Read the model definition and answer for the solid it produces. Units are mm, in the model's axes. A direction names the side the tool comes from. Give positions to 0.01 mm unless a question says otherwise; leave off trailing zeros. Write each loop counter-clockwise with the first axis right and the second up, starting at its lowest first coordinate (ties: lowest second). Pieces come first, ordered by that corner, then holes. Notation, with made-up numbers: M 10.5,46.5 L 52.5,46.5 A25 ccw 52.5,63.5 Z; hole C -2,70.5 d1. An arc over 180 degrees is marked long. Put each result on its own line as item: value.
from build123d import *

# Parameters (mm, degrees)
SKETCH1_W                               = 125
SKETCH1_H                               = 100
BOSS_EXTRUDE1_DEPTH                     = 15
SKETCH2_W                               = 75.5
SKETCH2_H                               = 45.5
CUT_EXTRUDE1_DEPTH                      = 5
FILLET1_R                               = 2.5
CHAMFER2_SIZE                           = 2.5
CBORE_FOR_M5_HEX_HEAD_BOLT1_D           = 5.5
CBORE_FOR_M5_HEX_HEAD_BOLT1_CBORE_D     = 12.24
CBORE_FOR_M5_HEX_HEAD_BOLT1_CBORE_DEPTH = 3.58
LPATTERN2_COUNT                         = 2
LPATTERN2_PITCH                         = 75
LPATTERN2_COUNT_DIR2                    = 2
LPATTERN2_PITCH_DIR2                    = 100
FILLET2_R                               = 2.5
CHAMFER3_SIZE                           = 2.5


with BuildPart() as part:
    # Sketch1 → Boss-Extrude1 (new body)
    with BuildSketch(Plane(origin=(0, 0, 0), x_dir=(1, 0, 0), z_dir=(0, 1, 0))):
        Rectangle(SKETCH1_W, SKETCH1_H)
    extrude(amount=BOSS_EXTRUDE1_DEPTH)

    # Sketch2 → Cut-Extrude1 (cut)
    with BuildSketch(Plane(origin=(0, 15, 0), x_dir=(1, 0, 0), z_dir=(0, 1, 0))):
        Rectangle(SKETCH2_W, SKETCH2_H)
    extrude(amount=-CUT_EXTRUDE1_DEPTH, mode=Mode.SUBTRACT)

    # Fillet1
    fillet1_edges = [part.edges().sort_by_distance(p)[0] for p in [
        (37.75, 12.5, -22.75),
        (37.75, 12.5, 22.75),
        (-37.75, 12.5, 22.75),
        (-37.75, 12.5, -22.75),
    ]]
    fillet(fillet1_edges, radius=FILLET1_R)

    # Chamfer2
    chamfer2_edges = [part.edges().sort_by_distance(p)[0] for p in [
        (0, 15, 22.75),
        (-37.75, 15, 0),
        (37.75, 15, 0),
        (0, 15, -22.75),
        (-37.017766953, 15, 22.017766953),
        (37.017766953, 15, 22.017766953),
        (37.017766953, 15, -22.017766953),
        (-37.017766953, 15, -22.017766953),
    ]]
    chamfer(chamfer2_edges, length=CHAMFER2_SIZE)

    # CBORE for M5 Hex Head Bolt1 (through all)
    with Locations(Plane(origin=(0, 15, 0), x_dir=(1, 0, 0), z_dir=(0, 1, 0))):
        with Locations((50, 37.5)):
            cbore_for_m5_hex_head_bolt1 = CounterBoreHole(CBORE_FOR_M5_HEX_HEAD_BOLT1_D / 2, CBORE_FOR_M5_HEX_HEAD_BOLT1_CBORE_D / 2, CBORE_FOR_M5_HEX_HEAD_BOLT1_CBORE_DEPTH)

    # LPattern2: CBORE for M5 Hex Head Bolt1 2 × 2
    with Locations(*[(-j * LPATTERN2_PITCH_DIR2, 0, i * LPATTERN2_PITCH) for i in range(LPATTERN2_COUNT) for j in range(LPATTERN2_COUNT_DIR2) if (i, j) != (0, 0)]):
        add(cbore_for_m5_hex_head_bolt1, mode=Mode.SUBTRACT)

    # Fillet2
    fillet2_edges = [part.edges().sort_by_distance(p)[0] for p in [
        (62.5, 7.5, 50),
        (-62.5, 7.5, 50),
        (-62.5, 7.5, -50),
        (62.5, 7.5, -50),
    ]]
    fillet(fillet2_edges, radius=FILLET2_R)

    # Chamfer3
    chamfer3_edges = [part.edges().sort_by_distance(p)[0] for p in [
        (-62.5, 15, 0),
        (0, 15, -50),
        (62.5, 15, 0),
        (0, 15, 50),
        (-61.767766953, 15, 49.267766953),
        (61.767766953, 15, 49.267766953),
        (61.767766953, 15, -49.267766953),
        (-61.767766953, 15, -49.267766953),
    ]]
    chamfer(chamfer3_edges, length=CHAMFER3_SIZE - 0.0001)  # a hair under: the kernel refuses the full size


solid = part.part
(1) For a pull along X with two mould halves and no side action, classify faces 3 (the face through (38.98, 13.73, 0.28)), 4 (the face through (-60.89, 13.73, 48.41)), 5 (the face through (60.89, 13.73, -48.41)) as +X half, -X half, draft (parallel to the pull), parting line (faces both ways), or undercut.
Result:
face 3: undercut
face 4: -X half
face 5: +X half
(2) Section A-A on z = 37.5 is taken. Determine the outline of the cut face in (x, y), and give its area (3 significant figures).
Result:
outline: M -62.5,0 L -52.75,0 L -52.75,11.42 L -56.12,11.42 L -56.12,15 L -60,15 L -62.5,12.5 Z; M -47.25,0 L 47.25,0 L 47.25,11.42 L 43.88,11.42 L 43.88,15 L -43.88,15 L -43.88,11.42 L -47.25,11.42 Z; M 52.75,0 L 62.5,0 L 62.5,12.5 L 60,15 L 56.12,15 L 56.12,11.42 L 52.75,11.42 Z
area: 1,660 mm²
(3) Section C-C on z = 4 is taken. Determine the outline of the cut face in (x, y), and give its area (4 significant figures).
Result:
outline: M -62.5,0 L 62.5,0 L 62.5,12.5 L 60,15 L 40.25,15 L 37.75,12.5 L 37.75,10 L -37.75,10 L -37.75,12.5 L -40.25,15 L -60,15 L -62.5,12.5 Z
area: 1,485 mm²
(4) Section B-B on x = -50 is taken. Determine the outline of the cut face in (y, z), and give its area (3 significant figures).
Result:
outline: M 0,-50 L 12.5,-50 L 15,-47.5 L 15,-43.62 L 11.42,-43.62 L 11.42,-40.25 L 0,-40.25 Z; M 0,-34.75 L 11.42,-34.75 L 11.42,-31.38 L 15,-31.38 L 15,31.38 L 11.42,31.38 L 11.42,34.75 L 0,34.75 Z; M 0,40.25 L 11.42,40.25 L 11.42,43.62 L 15,43.62 L 15,47.5 L 12.5,50 L 0,50 Z
area: 1,280 mm²
(5) Straight lines are drawn through the part: line 1 along Z through (x, y) = (50, 12.5); line 2 along X through (y, z) = (12.4, -37.5); line 3 along X through (y, z) = (6, -37.5). For each, find the intervals that lie inside material, in ascending order. Write a range as from..to.
Result:
line 1: z = -50..-43.62, -31.38..31.38, 43.62..50
line 2: x = -62.5..-56.12, -43.88..43.88, 56.12..62.5
line 3: x = -62.5..-52.75, -47.25..47.25, 52.75..62.5
(6) Which of the six approach directions +Z, -Z, +X, -X, +Y, -Y give full straight-line access (tool end or side, diameter ignored) to faces 1 (the face through (-62, 6, -49)), 2 (the face through (37.037, 11.232, -21.998))?
Result:
face 1: -Z, -X, +Y, -Y
face 2: +Y
(7) Given pin 1 Ø10 at (x, z) = (-50, 37.5) entering from +Y; pin 2 Ø10 at (x, z) = (49, 34.5) entering from +Y, each flat-ended and moving along its own axis, determine where each tip first touches the part or whether it passes through.
Result:
pin 1: stops at y = 11.42
pin 2: stops at y = 15
(8) Section D-D on x = -22.5 is taken. Determine the outline of the cut face in (y, z).
Result:
outline: M 0,-50 L 12.5,-50 L 15,-47.5 L 15,-25.25 L 12.5,-22.75 L 10,-22.75 L 10,22.75 L 12.5,22.75 L 15,25.25 L 15,47.5 L 12.5,50 L 0,50 Z
